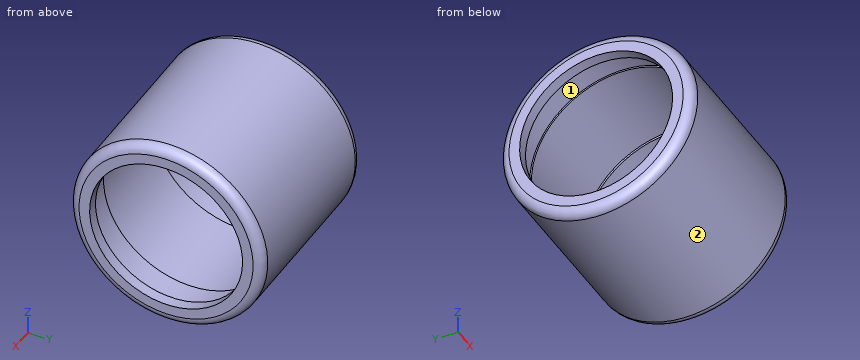
Autodesk Inventor part; units mm, degrees
ref_plane "YZ Plane" through (0, 0, 0) normal (1, 0, 0) x (0, 1, 0)
ref_plane "XZ Plane" through (0, 0, 0) normal (0, 1, 0) x (-1, 0, 0)
ref_plane "XY Plane" through (0, 0, 0) normal (0, 0, 1) x (1, 0, 0)
sketch "Sketch1" plane through (0, 0, 0) normal (0, 1, 0) x (-1, 0, 0)
  line L0 (1.975, 1.575) -> (7.2, 1.575)
  line L1 (1.8, 0) -> (1.8, 1.4)
  line L2 (0, 0) -> (1.8, 0)
  line L3 (0, 1.75) -> (0, 0)
  line L4 (28.425, 3.325) -> (1.575, 3.325)
  line L5 (30, 0) -> (30, 1.75)
  line L6 (28.2, 0) -> (30, 0)
  line L7 (28.2, 2.205) -> (28.2, 0)
  line L8 (22.8, 2.205) -> (27.71, 2.205)
  line L9 (22.8, 1.9285) -> (22.8, 2.205)
  line L10 (7.2, 1.9285) -> (22.8, 1.9285)
  line L11 (7.2, 1.575) -> (7.2, 1.9285)
  arc A0 (1.975, 1.575) -> (1.8, 1.4) centre (1.975, 1.4) ccw
  arc A1 (1.575, 3.325) -> (0, 1.75) centre (1.575, 1.75) ccw
  arc A2 (30, 1.75) -> (28.425, 3.325) centre (28.425, 1.75) ccw
  arc A3 (28.2, 2.205) -> (27.71, 2.205) centre (27.955, 2.205) ccw
  line L12 (30, -12.675) -> (0.4613, -12.675) construction
  point P0 (30, 0.875)
  dimension "d0" = 0
  dimension "d1" = 1.8
  dimension "d2" = 1.75
  dimension "d3" = 3.325
  dimension "d4" = 1.575
  dimension "d5" = 1.4
  dimension "d6" = 0.175
  dimension "d7" = 30
  dimension "d8" = 26.85
  dimension "d9" = 1.75
  dimension "d10" = 1.8
  dimension "d11" = 0.245
  dimension "d12" = 4.91
  dimension "d13" = 15.6
  dimension "d14" = 5.225
  dimension "d15" = 0.3535
  dimension "d16" = 0.2765
  dimension "d17" = 2.205
  dimension "d18" = 1.575
  dimension "d19" = 12.675
revolve "Revolution1" add sketch "Sketch1" angle 360 about axis through (-30, 0, -12.675) along (1, 0, 0)
properties part number "HFL2530_OutRing"
Here's how the part is built. I have some questions about the finished solid (model axes, mm). Face numbers are marked on the shaded views. Give positions to 0.01 mm unless a question says otherwise; leave off trailing zeros. Order: outer loops, then holes, each group sorted by start corner. A loop starts at its lowest first (then second) coordinate and runs counter-clockwise, first axis right, second up. Notation, with made-up numbers: (3, -28) - (52, -28) arc R21 ccw to (52, -15) - close; hole circle Ø2 at (68.5, 26). An arc over 180 degrees is marked (long way). Answer as a JSON object with one key per item and string values. Group by question number.
Item 1: Please list where these lines run through material, in increasing order: probe 1 along X at (y, z) = (-6.5, -24.5); probe 2 along Z at (x, y) = (-26.7, 0) (3 decimals); probe 3 along Z at (x, y) = (-24.5, 0.5).
Item 2: For P1, Ø5, axis at x = -6, y = 8, coming from the +Z side; P2, Ø2, axis at x = -15, y = -3.5, coming from the -Z side; P3, Ø2, axis at x = -12, z = -10.5, coming from the +Y side; P4, Ø8.5, axis at y = -2, z = -17, coming from the -X side, each with a flat end and sliding along its axis, tell me the tip position at first contact or that it passes through.
Item 3: If we section it at B-B on x = -8.5: Please give me the cut outline in (y, z) (1 decimal).
Item 4: If we section it at C-C on x = -4.5: Please give me the cut outline in (y, z) (3 decimals).
Item 5: If we mould it in two halves opening along X, with no side actions, what happens to the marked faces 1 and 2? For each: pulls with the +X half, pulls with the -X half, needs draft (parallel to the pull), parting line crosses it, or undercut.
Result set:
{
 "1": {"probe 1": "-30 to -28.2, -1.8 to 0", "probe 2": "-28.675 to -27.555, 2.205 to 3.325", "probe 3": "-28.67 to -27.55, 2.2 to 3.32"},
 "2": {"P1": "z = 2.35", "P2": "z = -28.48", "P3": "y = 15.96", "P4": "through"},
 "3": {"outline": "circle Ø32 at (0, -12.7); hole circle Ø29.2 at (0, -12.7)"},
 "4": {"outline": "circle Ø32 at (0, -12.675); hole circle Ø28.5 at (0, -12.675)"},
 "5": {"face 1": "undercut", "face 2": "needs draft"}
}
